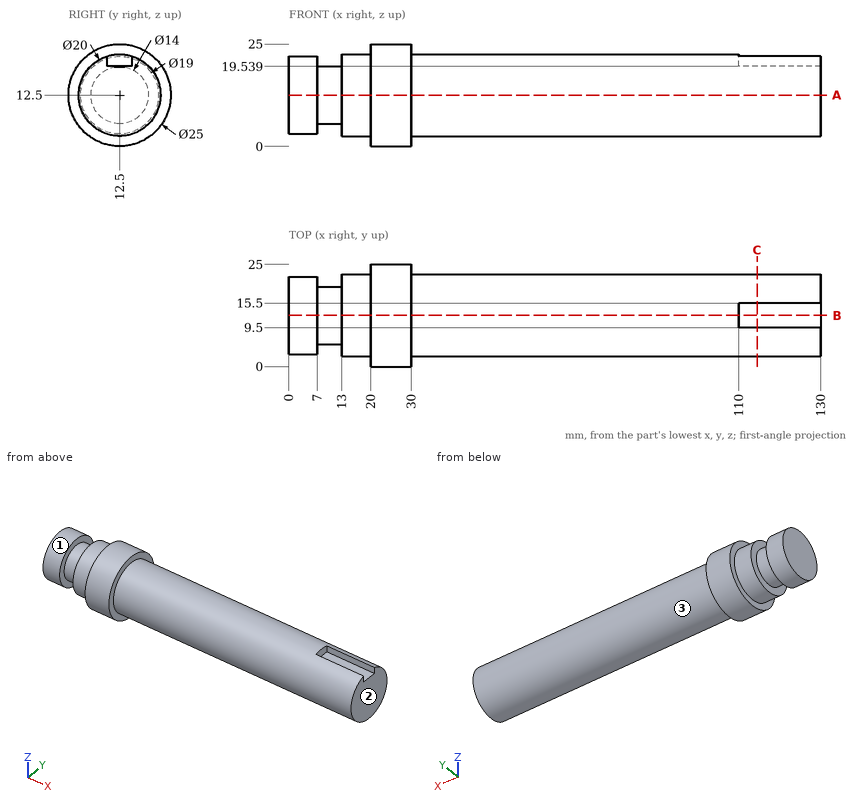
Geometry: see drawing. Coordinates: mm, zero at the bounding-box minimum. A direction names the side the tool comes from. Coordinates: 2 decimals unless noted, no trailing zeros. Loops run counter-clockwise (first coordinate to the right, second up) from the corner with the lowest first, then second, coordinate; pieces in that order, holes last. Notation, with made-up numbers: (4.25, 85) - (15.25, 85) arc R19 ccw to (15.25, 102) - close; hole circle Ø6 at (5, 4.5). An arc over 180 degrees is marked (long way). Put each result on its own line as item: value. Start each with the question number.
Q1. Cut plane A-A, the plane z = 12.5. Return loops of the section in (x, y).
Q2. Line query: line 1 (X direction, y = 8.25, z = 18.25); line 2 (X direction, y = 9.5, z = 23); line 3 (X direction, y = 6, z = 19.75). Output: solid intervals per line, ascending.
Q3. Cut plane C-C, the plane x = 114.5. Return loops of the section in (y, z), and give its area (3 significant figures).
Q4. Set-up query: the marked faces 1, 2 and 3. Return all of +Z, -Z, +X, -X, +Y, -Y with unobstructed straight access to the full face (end or side cutting, diameter ignored); none if empty.
Q5. Cut plane B-B, the plane y = 12.5. Return loops of the section in (x, z), and give its area (3 significant figures).
Q6. Pin query (flat end, axial travel): pin 1 Ø5 at (x, y) = (52.5, 17) entering from -Z; pin 2 Ø10 at (y, z) = (8.5, 16) entering from -X; pin 3 Ø1.2 at (x, z) = (121, 20.5) entering from +Y (1 decimal); pin 4 Ø3 at (x, z) = (86.5, 16) entering from -Y. Return the tip coordinate at first contact, or that it passes through.
Filled sheet:
1. outline: (0, 3) - (7, 3) - (7, 5.5) - (13, 5.5) - (13, 2.5) - (20, 2.5) - (20, 0) - (30, 0) - (30, 2.5) - (130, 2.5) - (130, 22.5) - (30, 22.5) - (30, 25) - (20, 25) - (20, 22.5) - (13, 22.5) - (13, 19.5) - (7, 19.5) - (7, 22) - (0, 22) - close
2. line 1: 0 to 7, 13 to 130
2. line 2: 20 to 30
2. line 3: 13 to 130
3. outline: (9.5, 19.54) - (9.5, 22.04) arc R10 ccw (long way) to (15.5, 22.04) - (15.5, 19.54) - close
3. area: 297 mm²
4. face 1: -X
4. face 2: +Z, -Z, +X, +Y, -Y
4. face 3: +X
5. outline: (0, 3) - (7, 3) - (7, 5.5) - (13, 5.5) - (13, 2.5) - (20, 2.5) - (20, 0) - (30, 0) - (30, 2.5) - (130, 2.5) - (130, 19.54) - (110, 19.54) - (110, 22.5) - (30, 22.5) - (30, 25) - (20, 25) - (20, 22.5) - (13, 22.5) - (13, 19.5) - (7, 19.5) - (7, 22) - (0, 22) - close
5. area: 2,550 mm²
6. pin 1: z = 2.7
6. pin 2: x = 0
6. pin 3: y = 19.2
6. pin 4: y = 2.7
